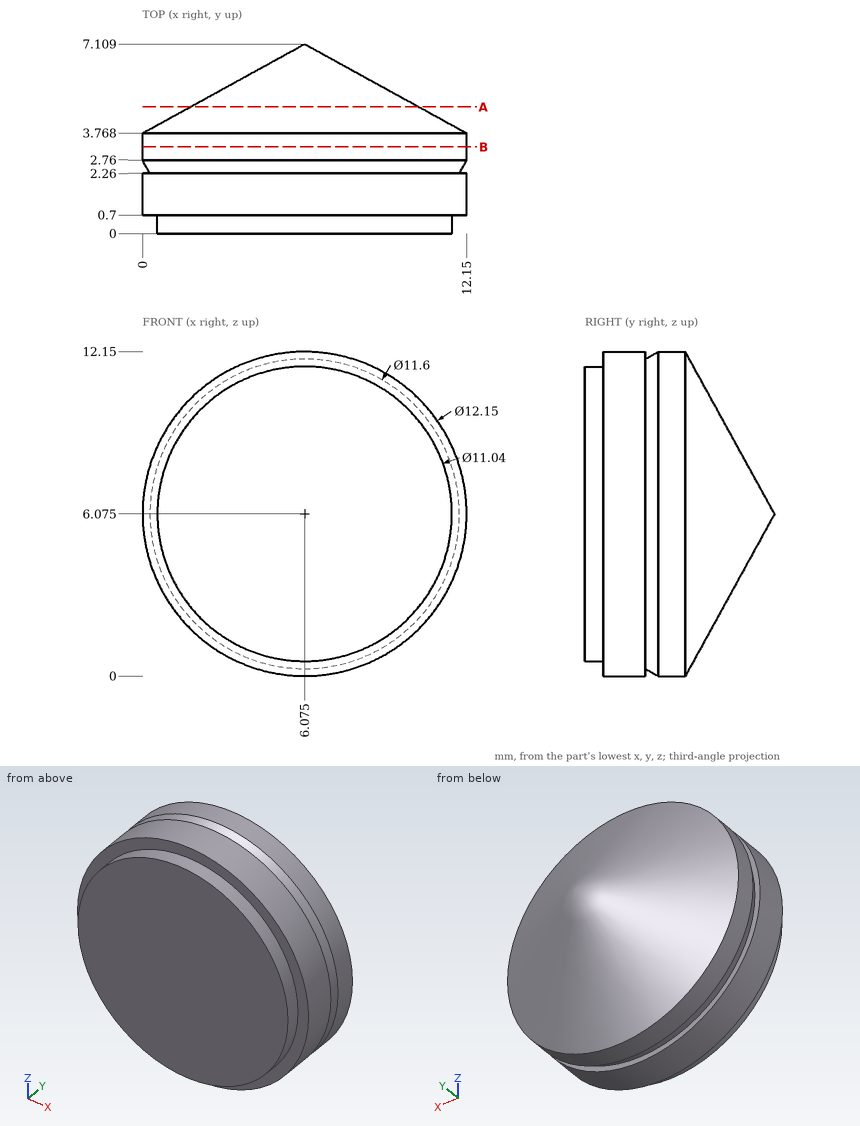
Geometry: see drawing. Coordinates: mm, zero at the bounding-box minimum. Round coordinates to 2 decimals unless told otherwise and drop trailing zeros. Loops run counter-clockwise (first coordinate to the right, second up) from the corner with the lowest first, then second, coordinate; pieces in that order, holes last. Notation, with made-up numbers: (9, 35) -> (49, 35) arc R21 cw to (49, 41) -> close; hole circle Ø2 at (8, 69.25). An arc over 180 degrees is marked (long way). Use one line per item in the form item = value. Start each with the question number.
Item 1: Section query B-B on y = 3.25. Return the cut outline in (x, z) (3 decimals).
Item 2: Material intervals for L1, parallel to Z at x = 6.25, y = 2; L2, parallel to Y at x = 10, z = 1.5 (1 decimal); L3, parallel to Y at x = 5.75, z = 4.5 (1 decimal), sorted ascending. Write a range as from..to.
Item 3: Contact query for flat-ended pins moving along their axis: pin 1 Ø6 at (x, z) = (8.5, 2) entering from +Y; pin 2 Ø2 at (x, z) = (7.5, 5.5) entering from +Y; pin 3 Ø3 at (x, z) = (2, 4) entering from +Y. Output: stop coordinate, or through.
Item 4: Section query A-A on y = 4.75. Return the cut outline in (x, z) (1 decimal), then the cut area to 3 significant figures.
Ans:
q1.outline = circle Ø12.15 at (6.075, 6.075)
q2.L1 = 0..12.15
q2.L2 = 0.7..2.3, 2.7..3.8
q2.L3 = 0..6.2
q3.pin_1 = 6.15
q3.pin_2 = 6.81
q3.pin_3 = 5.42
q4.outline = circle Ø8.6 at (6.1, 6.1)
q4.area = 57.8 mm^2
